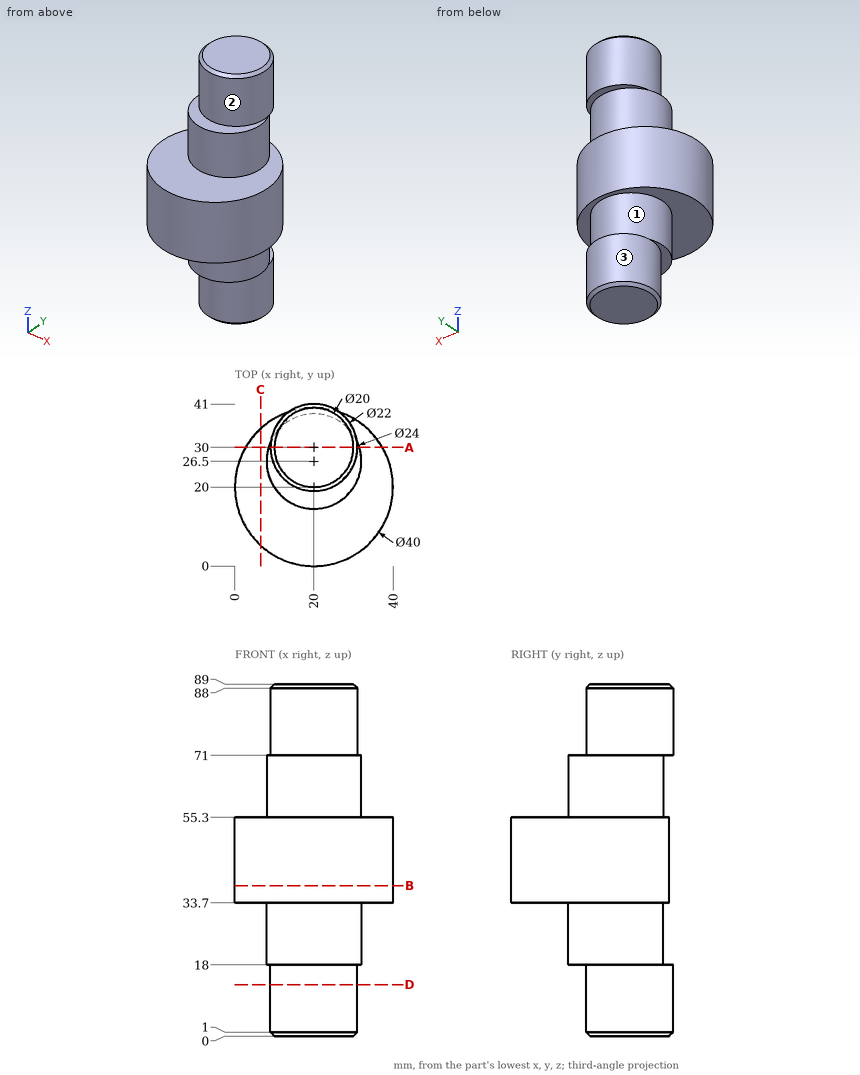
Print and shaded views of the part. All mm, measured from the part's lowest x, y and z. A direction names the side the tool comes from. Give positions to 0.01 mm unless a question says otherwise; leave off trailing zeros. Order: outer loops, then holes, each group sorted by start corner. A loop starts at its lowest first (then second) coordinate and runs counter-clockwise, first axis right, second up. Notation, with made-up numbers: (74, 86) - (117, 86) arc R21 cw to (117, 114) - close; hole circle Ø3 at (62.5, 85). An arc over 180 degrees is marked (long way). Use a Markdown table: item, result.
1) Saw through at D-D on z = 13. List the corners of the cut face in (x, y), plus the area to 3 significant figures.
Checked values:
| item | result |
|---|---|
| outline | circle Ø22 at (20, 30) |
| area | 380 mm² |
2) Flat gauge pins, fed straight in: P1, Ø2, axis at x = 29, z = 76.5, coming from the -Y side; P2, Ø5, axis at x = 16, y = 24, coming from the -Z side; P3, Ø10, axis at x = 15.5, y = 12, coming from the -Z side; P4, Ø6, axis at x = 27, y = 14.5, coming from the +Z side. Where does each tip first touch, or does it go through?
Checked values:
| item | result |
|---|---|
| P1 | y = 22.45 |
| P2 | z = 0 |
| P3 | z = 18 |
| P4 | z = 71 |
3) Saw through at B-B on z = 38. List the corners of the cut face in (x, y).
Checked values:
| item | result |
|---|---|
| outline | circle Ø40 at (20, 20) |
4) Saw through at C-C on x = 6.5. List the corners of the cut face in (y, z), plus the area to 3 significant figures.
Checked values:
| item | result |
|---|---|
| outline | (5.24, 33.7) - (34.76, 33.7) - (34.76, 55.3) - (5.24, 55.3) - close |
| area | 637 mm² |
5) Saw through at A-A on y = 30. List the corners of the cut face in (x, z).
Checked values:
| item | result |
|---|---|
| outline | (2.68, 33.7) - (8.52, 33.7) - (8.52, 18) - (9, 18) - (9, 1) - (10, 0) - (30, 0) - (31, 1) - (31, 18) - (31.48, 18) - (31.48, 33.7) - (37.32, 33.7) - (37.32, 55.3) - (31.48, 55.3) - (31.48, 71) - (31, 71) - (31, 88) - (30, 89) - (10, 89) - (9, 88) - (9, 71) - (8.52, 71) - (8.52, 55.3) - (2.68, 55.3) - close |
6) Probe L1, parallel to Z at x = 5, y = 21; L2, parallel to X at y = 31.5, z = 66.5; L3, parallel to X at y = 28, z = 16.5. List the from-to ranges inside material, lowest first. Write a range as from..to.
Checked values:
| item | result |
|---|---|
| L1 | 33.7..55.3 |
| L2 | 9.09..30.91 |
| L3 | 9.18..30.82 |
7) 3-axis set-ups, long thin cutter, end or side, ignore diameter. For the marked faces 1, 2 and 3: which of +Z, -Z, +X, -X, +Y, -Y reach the whole face in a straight line?
Checked values:
| item | result |
|---|---|
| face 1 | none |
| face 2 | +Z |
| face 3 | -Z |
